Geometry check sheet. Reference: the model listing, model coordinates, mm. Face numbers are marked on the shaded views. A direction names the side the tool comes from. Round coordinates to 2 decimals unless told otherwise and drop trailing zeros. Order: outer loops, then holes, each group sorted by start corner. A loop starts at its lowest first (then second) coordinate and runs counter-clockwise, first axis right, second up. Notation, with made-up numbers: (78, 82.25) -> (102, 82.25) arc R19 ccw to (102, 101.25) -> close; hole circle Ø9 at (-15, -11). An arc over 180 degrees is marked (long way). Use a Markdown table: item, result. Add a question column.
Item 1: Material ranges on probe 1 along Z at (x, y) = (2.4, 0); probe 2 along Z at (x, y) = (5.25, 0); probe 3 along Z at (x, y) = (5, 2.2), recorded low to high. Write a range as [from, to].
Item 2: Sectioned sample at D-D, the plane x = 0.75. Record the cut outline in (y, z).
Item 3: Sectioned sample at C-C, the plane x = 4.5. Record the cut outline in (y, z), and give its area (3 significant figures).
Item 4: Set-up check for the marked faces 1, 2 and 3: record each of +Z, -Z, +X, -X, +Y, -Y from which the full face is reachable in a straight line by a thin tool's end or side.
Item 5: Sectioned sample at B-B, the plane y = 0. Record the cut outline in (x, z).
Item 6: Gauge pin test, flat ends, axial feed: pin 1 Ø1.9 at (y, z) = (0, 50) entering from +X; pin 2 Ø2 at (x, y) = (4.5, 0) entering from -Z. Record the tip position at first contact, or that the pin passes through.
Item 7: Sectioned sample at A-A, the plane z = 25. Record the cut outline in (x, y).
from build123d import *

# Parameters (mm, degrees)
F0_R     = 1.55
F0_W     = 5
F0_H     = 4
F1_DEPTH = 3
F2_DEPTH = 7.2


with BuildPart() as f1:
    # F0 (on Right) → F1 (new body)
    with BuildSketch(Plane.YZ):
        with BuildLine():
            Line((-2.5, 50), (-2.5, 27))
            Line((-2.5, 27), (2.5, 27))
            Line((2.5, 27), (2.5, 50))
            ThreePointArc((2.5, 50), (0, 52.5), (-2.5, 50))
        make_face()
        with Locations((0, 50)):
            Circle(F0_R, mode=Mode.SUBTRACT)
        with Locations((0, 25)):
            Rectangle(F0_W, F0_H)
        with Locations((0, 25)):
            Circle(F0_R, mode=Mode.SUBTRACT)
        with BuildLine():
            Line((-2.5, 23), (-2.5, 0))
            ThreePointArc((-2.5, 0), (0, -2.5), (2.5, 0))
            Line((2.5, 0), (2.5, 23))
            Line((2.5, 23), (-2.5, 23))
        make_face()
        Circle(F0_R, mode=Mode.SUBTRACT)
    extrude(amount=F1_DEPTH)

    # F0 (on Right) → F2 (join)
    with BuildSketch(Plane.YZ):
        with Locations((0, 25)):
            Rectangle(F0_W, F0_H)
        with Locations((0, 25)):
            Circle(F0_R, mode=Mode.SUBTRACT)
    extrude(amount=F2_DEPTH)


solid = f1.part
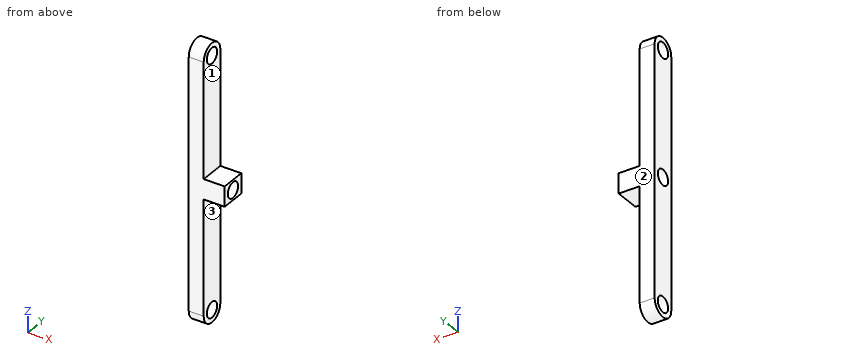
Found:
| question | item | result |
|---|---|---|
| 1 | probe 1 | z = [-2.5, -1.55], [1.55, 23.45], [26.55, 48.45], [51.55, 52.5] |
| 1 | probe 2 | z = [23, 23.45], [26.55, 27] |
| 1 | probe 3 | z = [23, 27] |
| 2 | outline | (-2.5, 0) arc R2.5 ccw to (2.5, 0) -> (2.5, 50) arc R2.5 ccw to (-2.5, 50) -> close; hole circle Ø3.1 at (0, 0); hole circle Ø3.1 at (0, 25); hole circle Ø3.1 at (0, 50) |
| 3 | outline | (-2.5, 23) -> (2.5, 23) -> (2.5, 27) -> (-2.5, 27) -> close; hole circle Ø3.1 at (0, 25) |
| 3 | area | 12.5 mm2 |
| 4 | face 1 | +Z, +X, +Y, -Y |
| 4 | face 2 | +Z, -Z, +X, -X, +Y |
| 4 | face 3 | -Z, +X, +Y, -Y |
| 5 | outline | (0, -2.5) -> (3, -2.5) -> (3, -1.55) -> (0, -1.55) -> close; (0, 1.55) -> (3, 1.55) -> (3, 23) -> (7.2, 23) -> (7.2, 23.45) -> (0, 23.45) -> close; (0, 26.55) -> (7.2, 26.55) -> (7.2, 27) -> (3, 27) -> (3, 48.45) -> (0, 48.45) -> close; (0, 51.55) -> (3, 51.55) -> (3, 52.5) -> (0, 52.5) -> close |
| 6 | pin 1 | passes through |
| 6 | pin 2 | stops at z = 23 |
| 7 | outline | (0, -2.5) -> (7.2, -2.5) -> (7.2, -1.55) -> (0, -1.55) -> close; (0, 1.55) -> (7.2, 1.55) -> (7.2, 2.5) -> (0, 2.5) -> close |
